Source: three-view drawing plus pictorial views. Frame: mm from the lowest corner of the part. A direction names the side the tool comes from. Round coordinates to 2 decimals unless told otherwise and drop trailing zeros. Write each loop counter-clockwise with the first axis right and the second up, starting at its lowest first coordinate (ties: lowest second). Pieces come first, ordered by that corner, then holes. Notation, with made-up numbers: M 27.5,59.5 L 50.5,59.5 A22 ccw 50.5,97.5 Z; hole C 78.5,18.5 d11. An arc over 180 degrees is marked long. Answer as CSV lines item,"result". Start each with the question number.
Q1. Section query A-A on x = 92. Output: boundary loops of the cut face in (y, z).
Q2. Ray query, probe 1 along Y at (x, z) = (445.77, 4) (3 decimals); probe 2 along Z at (x, y) = (58, 8.5); probe 3 along X at (y, z) = (12.5, 6.5). Return the intervals inside material, ascending.
Q3. Section query B-B on z = 9.25. Output: boundary loops of the cut face in (x, y).
Q4. Reachability of the marked faces 1 and 2 from +Z, -Z, +X, -X, +Y, -Y: full face, straight path, thin tool, end or side. Return the list, or none.
Q5. First-contact query: pin 1 (9 mm diameter, centred on x = 445.77, y = 30.988, fed in from +Z). Flat tip, straight axial feed; report the tip coordinate or a pass-through.
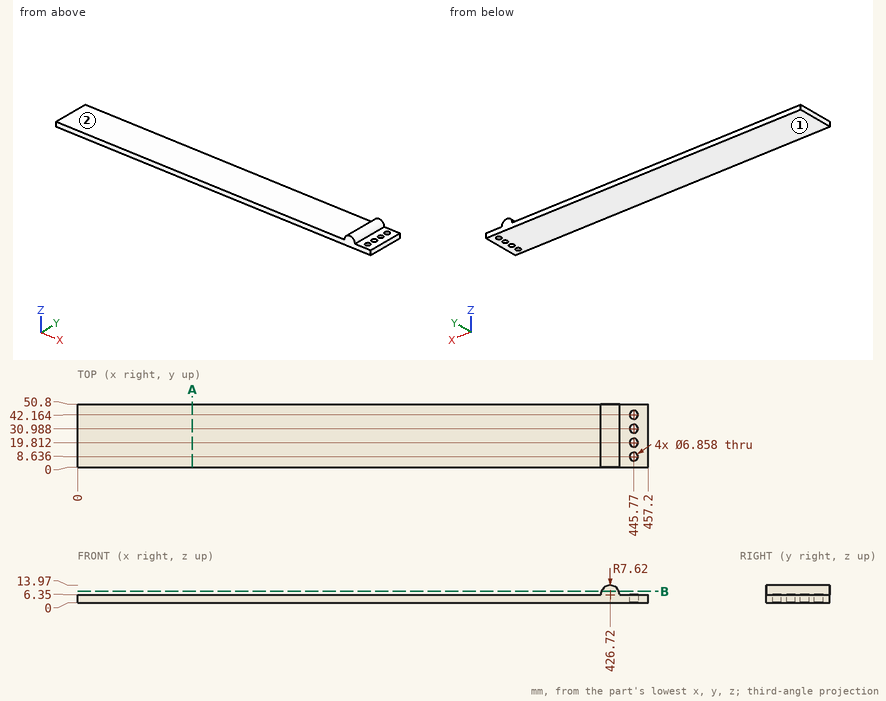
Entries:
1,outline,"M 0,0 L 50.8,0 L 50.8,6.35 L 0,6.35 Z"
2,probe 1,"y = 0 to 5.207, 12.065 to 16.383, 23.241 to 27.559, 34.417 to 38.735, 45.593 to 50.8"
2,probe 2,"z = 0 to 6.35"
2,probe 3,"x = 419.1 to 434.34"
3,outline,"M 419.67,0 L 433.77,0 L 433.77,50.8 L 419.67,50.8 Z"
4,face 1,"-Z, +X, -X, +Y, -Y"
4,face 2,"+Z, -X, +Y, -Y"
5,pin 1,"stops at z = 6.35"
